Design review of the part shown in the three views and the two pictorial views. Dimensions are in mm from the part's minimum x, y and z. Give positions to 0.01 mm unless a question says otherwise; leave off trailing zeros. Write each loop counter-clockwise with the first axis right and the second up, starting at its lowest first coordinate (ties: lowest second). Pieces come first, ordered by that corner, then holes. Notation, with made-up numbers: M 20.25,67.25 L 40.25,67.25 A16 cw 40.25,89.25 Z; hole C 73.5,84.5 d4. An arc over 180 degrees is marked long. Write item = value, one per line.
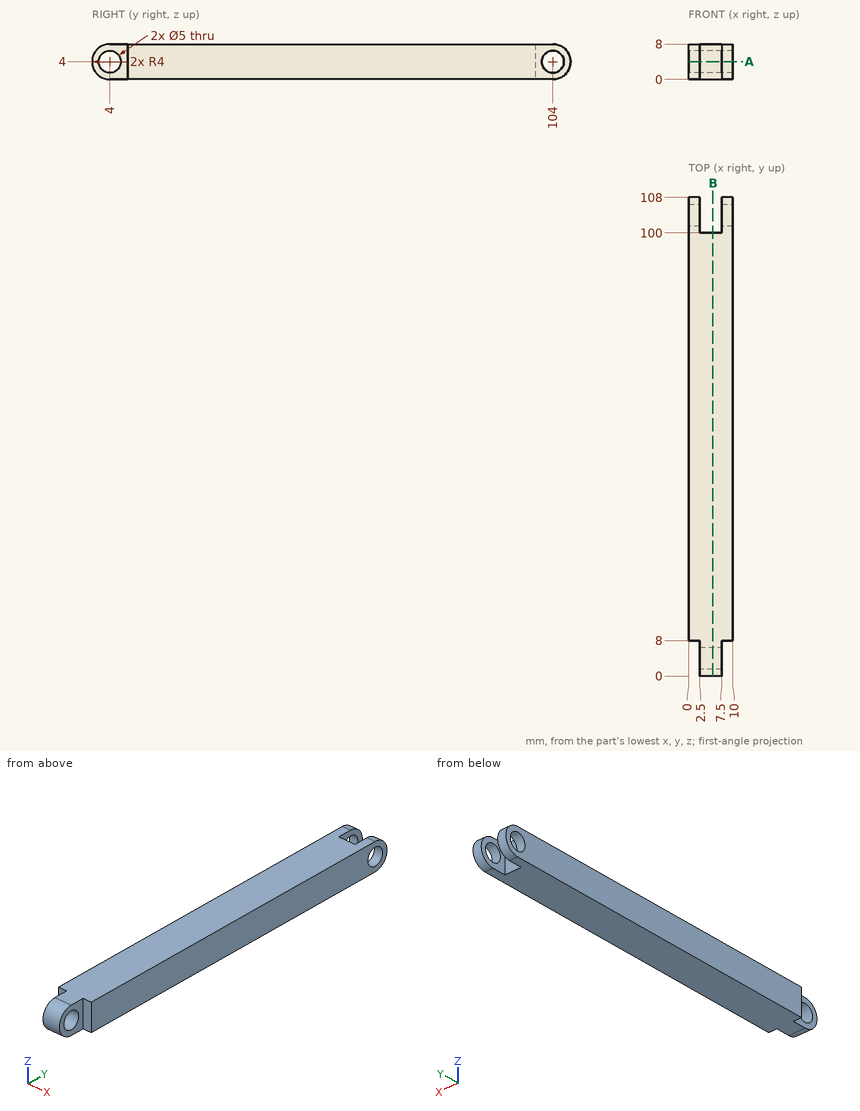
1. For line 1 along Z through (x, y) = (5.8, 4); line 2 along Y through (x, z) = (1.05, 4); line 3 along Y through (x, z) = (5.35, 4), list the stretches that pass through material, from the lowest coordinate up. Write a range as from..to.
Responses:
line_1 = 0..1.5, 6.5..8
line_2 = 8..101.5, 106.5..108
line_3 = 0..1.5, 6.5..100
2. We need section B-B, the plane x = 5.5. Write out the cut boundary in (y, z).
Responses:
outline = M 4,0 L 100,0 L 100,8 L 4,8 A4 ccw Z; hole C 4,4 d5
3. Insertion check: P1, Ø4, axis at y = 104, z = 4, coming from the +X side; P2, Ø1, axis at x = 5.5, z = 6, coming from the -Y side; P3, Ø4, axis at x = 8.5, z = 6, coming from the -Y side; P4, Ø1.2, axis at x = 1.5, z = 5.5, coming from the -Y side. Each pin has a flat end and moves straight along its axis. Give the tip position at first contact, or say it passes through.
Responses:
P1 = through
P2 = 0.29
P3 = 0.01
P4 = 8
4. We need section A-A, the plane z = 4. Write out the cut boundary in (x, y), then the cut area to 3 significant figures.
Responses:
outline = M 0,8 L 2.5,8 L 2.5,6.5 L 7.5,6.5 L 7.5,8 L 10,8 L 10,101.5 L 7.5,101.5 L 7.5,100 L 2.5,100 L 2.5,101.5 L 0,101.5 Z; M 0,106.5 L 2.5,106.5 L 2.5,108 L 0,108 Z; M 2.5,0 L 7.5,0 L 7.5,1.5 L 2.5,1.5 Z; M 7.5,106.5 L 10,106.5 L 10,108 L 7.5,108 Z
area = 950 mm2
